The listing builds one solid part. Answer for the finished solid, in the listing's coordinates (mm). A direction names the side the tool comes from. Give positions to 0.01 mm unless a question says otherwise; leave off trailing zeros. Write each loop counter-clockwise with the first axis right and the second up, starting at its lowest first coordinate (ties: lowest second). Pieces come first, ordered by that corner, then holes. Notation, with made-up numbers: M 50,-32.75 L 97,-32.75 A14 cw 97,-15.75 Z; hole C 33.25,54.5 d6. An arc over 180 degrees is marked long. Return JSON: item names as keys, results as strings.
from build123d import *

# Parameters (mm, degrees)
BOSS_EXTRUDE2_DEPTH = 9.525
SKETCH3_R           = 6.35
CUT_EXTRUDE2_DEPTH  = 19.05


with BuildPart() as part:
    # Sketch1 → Boss-Extrude2 (new, symmetric)
    with BuildSketch(Plane.XY):
        with BuildLine():
            Line((-25.4, 71.842048969), (-25.4, 65.492048969))
            Line((-25.4, 65.492048969), (25.4, 65.492048969))
            Line((25.4, 65.492048969), (25.4, 71.842048969))
            ThreePointArc((25.4, 71.842048969), (53.881536726, 53.881536726), (71.842048969, 25.4))
            Line((71.842048969, 25.4), (65.492048969, 25.4))
            Line((65.492048969, 25.4), (65.492048969, -25.4))
            Line((65.492048969, -25.4), (71.842048969, -25.4))
            ThreePointArc((71.842048969, -25.4), (53.881536726, -53.881536726), (25.4, -71.842048969))
            Line((25.4, -71.842048969), (25.4, -65.492048969))
            Line((25.4, -65.492048969), (-25.4, -65.492048969))
            Line((-25.4, -65.492048969), (-25.4, -71.842048969))
            ThreePointArc((-25.4, -71.842048969), (-53.881536726, -53.881536726), (-71.842048969, -25.4))
            Line((-71.842048969, -25.4), (-65.492048969, -25.4))
            Line((-65.492048969, -25.4), (-65.492048969, 25.4))
            Line((-65.492048969, 25.4), (-71.842048969, 25.4))
            ThreePointArc((-71.842048969, 25.4), (-53.881536726, 53.881536726), (-25.4, 71.842048969))
        make_face()
    extrude(amount=BOSS_EXTRUDE2_DEPTH, both=True)

    # Sketch3 → Cut-Extrude2 (cut)
    with BuildSketch(Plane.XY.offset(9.525)):
        Circle(SKETCH3_R)
    extrude(amount=-CUT_EXTRUDE2_DEPTH, mode=Mode.SUBTRACT)


solid = part.part
Item 1: A cutting plane is placed at C-C, the plane z = 2.25. Write down the section's boundary in (x, y), plus the area to 3 significant figures.
Geometry results:
{"outline": "M -71.84,-25.4 A76.2 ccw -25.4,-71.84 L -25.4,-65.49 L 25.4,-65.49 L 25.4,-71.84 A76.2 ccw 71.84,-25.4 L 65.49,-25.4 L 65.49,25.4 L 71.84,25.4 A76.2 ccw 25.4,71.84 L 25.4,65.49 L -25.4,65.49 L -25.4,71.84 A76.2 ccw -71.84,25.4 L -65.49,25.4 L -65.49,-25.4 Z; hole C 0,0 d12.7", "area": "16,200 mm2"}
Item 2: Which of the six approach directions +Z, -Z, +X, -X, +Y, -Y give full straight-line access (tool end or side, diameter ignored) to faces 1 (the flat face through (-69, -25.4, 0)), 2 (the cylindrical face through (-54.22, 53.54, 0.13)), 3 (the flat face through (0, -65.492, 0)), 4 (the flat face through (69, 25.4, 0)), 5 (the flat face through (25.4, 69, 0))?
Geometry results:
{"face 1": "+Z, -Z, -X", "face 2": "+Z, -Z, -X, +Y", "face 3": "+Z, -Z, -Y", "face 4": "+Z, -Z, +X", "face 5": "+Z, -Z, +Y"}
Item 3: A cutting plane is placed at D-D, the plane y = -37. Write down the section's boundary in (x, z) (3 decimals).
Geometry results:
{"outline": "M -66.614,-9.525 L 66.614,-9.525 L 66.614,9.525 L -66.614,9.525 Z"}
Item 4: A cutting plane is placed at A-A, the plane x = 0. Write down the section's boundary in (y, z) (3 decimals).
Geometry results:
{"outline": "M -65.492,-9.525 L -6.35,-9.525 L -6.35,9.525 L -65.492,9.525 Z; M 6.35,-9.525 L 65.492,-9.525 L 65.492,9.525 L 6.35,9.525 Z"}
Item 5: Find the intervals of material crossed by line 1 (Y direction, x = 0, z = -3.75); line 2 (Y direction, x = 12, z = -1.5); line 3 (X direction, y = 39, z = 7.75), in increasing order.
Geometry results:
{"line 1": "y = -65.49 to -6.35, 6.35 to 65.49", "line 2": "y = -65.49 to 65.49", "line 3": "x = -65.46 to 65.46"}
Item 6: Given pin 1 Ø10 at (y, z) = (-0.5, -5.5) entering from -X; pin 2 Ø7 at (y, z) = (-67.5, 3) entering from -X; pin 3 Ø5 at (y, z) = (-67.5, -2) entering from +X, each flat-ended and moving along its own axis, determine where each tip first touches the part or whether it passes through.
Geometry results:
{"pin 1": "stops at x = -65.49", "pin 2": "stops at x = -41.36", "pin 3": "stops at x = 39.77"}
Item 7: Determine the mould class of faces 6 (the cylindrical face through (-53.54, -54.22, 0.13)), 7 (the flat face through (69, -25.4, 0)), 8 (the flat face through (65.492, 0, 0)), 9 (the flat face through (-15, 1, -9.525)) for opening direction Y: +Y half, -Y half, draft (parallel to the pull), parting line (faces both ways), or undercut.
Geometry results:
{"face 6": "-Y half", "face 7": "undercut", "face 8": "undercut", "face 9": "draft"}
